For this review, use the dimensioned drawing (mm, ordinates from the lowest corner) and the shaded views. A direction names the side the tool comes from. Round coordinates to 2 decimals unless told otherwise and drop trailing zeros. Loops run counter-clockwise (first coordinate to the right, second up) from the corner with the lowest first, then second, coordinate; pieces in that order, holes last. Notation, with made-up numbers: M 6,60.5 L 55,60.5 A11 cw 55,65.5 Z; hole C -15,70 d3. An arc over 180 degrees is marked long. Answer as a JSON object with one key per item and string values. Group by question number.
Item 1: Consider section A-A (z = 26). Give the boundary of the cut face in (x, y).
Item 2: Tool access review of the marked faces 1, 2 and 3: name each direction out of +Z, -Z, +X, -X, +Y, -Y from which nothing blocks a thin tool from reaching the whole face with its end or side.
Item 3: Consider section B-B (y = 16.5). Give the boundary of the cut face in (x, z), and give its area (3 significant figures).
Item 4: Insertion check: P1, Ø1.5, axis at x = 35, z = 72.5, coming from the +Y side; P2, Ø5, axis at x = 23.5, z = 34.5, coming from the -Y side; P3, Ø12, axis at x = 16, z = 17, coming from the -Y side. Each pin has a flat end and moves straight along its axis. Give the tip position at first contact, or say it passes through.
Item 5: Consider section C-C (x = 28). Give the boundary of the cut face in (y, z).
Item 6: To check wall thickness, follow line 1 (Y direction, x = 83, z = 13.5); line 2 (X direction, y = 59, z = 34); line 3 (X direction, y = 14.5, z = 68) (1 decimal). State the ranges of each line that lie inside material, in increasing order.
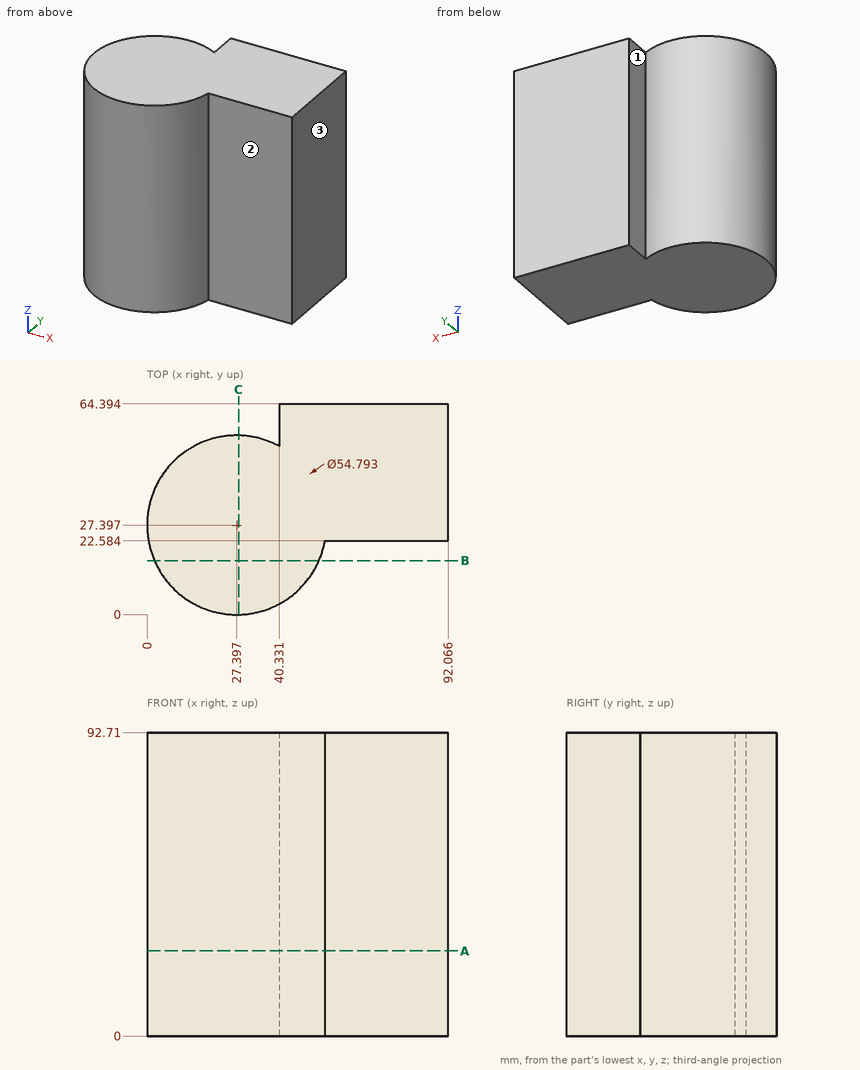
Geometry results:
{
 "1": {"outline": "M 40.33,51.55 A27.4 ccw long 54.37,22.58 L 92.07,22.58 L 92.07,64.39 L 40.33,64.39 Z"},
 "2": {"face 1": "+Z, -Z, +Y", "face 2": "+Z, -Z, +X, -Y", "face 3": "+Z, -Z, +X, +Y, -Y"},
 "3": {"outline": "M 2.26,0 L 52.53,0 L 52.53,92.71 L 2.26,92.71 Z", "area": "4,660 mm^2"},
 "4": {"P1": "stops at y = 53.92", "P2": "stops at y = 0.04", "P3": "stops at y = 0.54"},
 "5": {"outline": "M 0.01,0 L 54.79,0 L 54.79,92.71 L 0.01,92.71 Z"},
 "6": {"line 1": "y = 22.58 to 64.39", "line 2": "x = 40.33 to 92.07", "line 3": "x = 3.2 to 51.6"}
}
